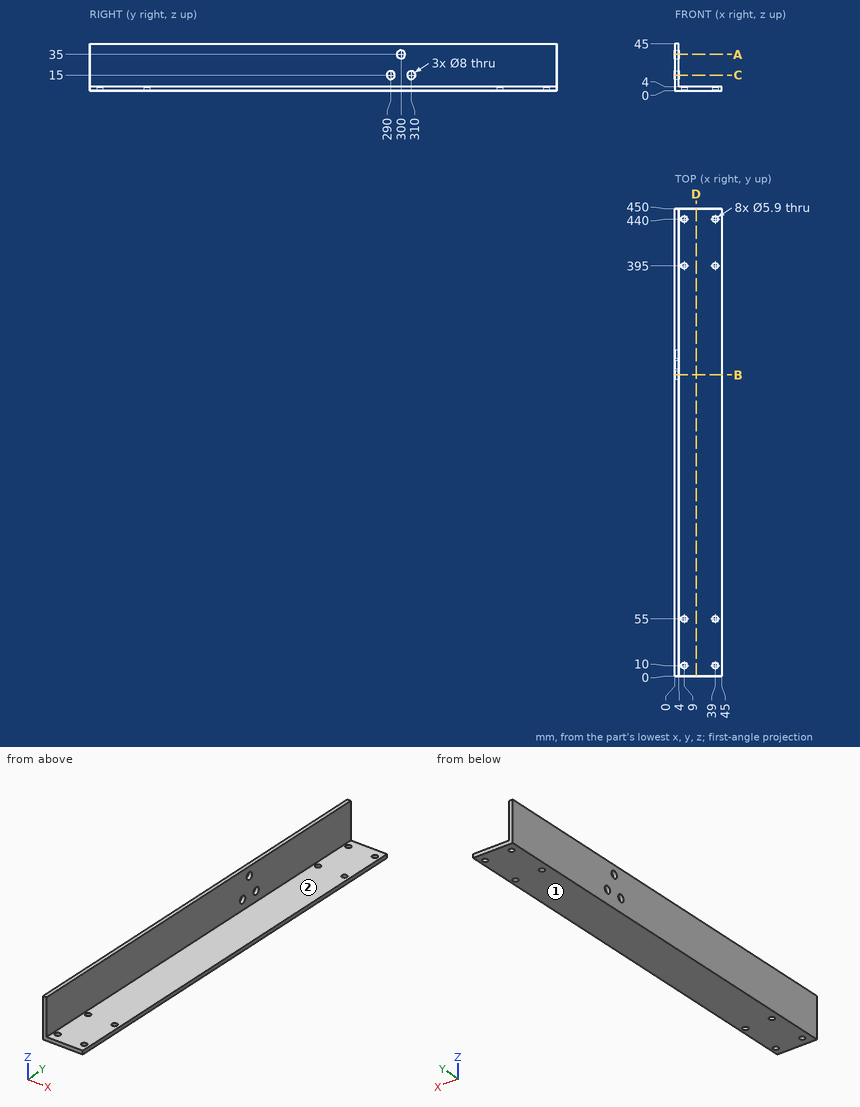
Part print with two shaded views. Sizes in mm from the minimum x, y, z corner. A direction names the side the tool comes from. Coordinates: 2 decimals unless noted, no trailing zeros. Order: outer loops, then holes, each group sorted by start corner. A loop starts at its lowest first (then second) coordinate and runs counter-clockwise, first axis right, second up.
(1) Drill centre lines: L1, parallel to Y at x = 9, z = 3; L2, parallel to Y at x = 38, z = 2; L3, parallel to X at y = 79, z = 21. Where is each one in solid material? Low to high.
Solution:
L1: y = 0 to 7.05, 12.95 to 52.05, 57.95 to 392.05, 397.95 to 437.05, 442.95 to 450
L2: y = 0 to 7.22, 12.78 to 52.22, 57.78 to 392.22, 397.78 to 437.22, 442.78 to 450
L3: x = 0 to 4
(2) Saw through at B-B, the plane y = 290. Write the cut outline in (x, z), and give its area (3 significant figures).
Solution:
outline: (0, 0) - (45, 0) - (45, 4) - (4, 4) - (4, 11) - (0, 11) - close; (0, 19) - (4, 19) - (4, 45) - (0, 45) - close
area: 312 mm2
(3) Pin check, flat tips, straight feed: pin 1 Ø8 at (y, z) = (400.5, 20.5) entering from +X; pin 2 Ø12.5 at (x, y) = (18.5, 241.5) entering from +Z; pin 3 Ø6 at (x, y) = (11.5, 82) entering from -Z. Stop position of each tip, or through.
Solution:
pin 1: stops at x = 4
pin 2: stops at z = 4
pin 3: stops at z = 0
(4) Saw through at A-A, the plane z = 35. Write the cut outline in (x, y), and give its area (3 significant figures).
Solution:
outline: (0, 0) - (4, 0) - (4, 296) - (0, 296) - close; (0, 304) - (4, 304) - (4, 450) - (0, 450) - close
area: 1,770 mm2
(5) Saw through at C-C, the plane z = 15. Write the cut outline in (x, y), and give its area (3 significant figures).
Solution:
outline: (0, 0) - (4, 0) - (4, 286) - (0, 286) - close; (0, 294) - (4, 294) - (4, 306) - (0, 306) - close; (0, 314) - (4, 314) - (4, 450) - (0, 450) - close
area: 1,740 mm2
(6) Which spindle directions (+Z, -Z, +X, -X, +Y, -Y) get a long thin tool onto all of the face, cutting with end or side? Do the marked faces 1 and 2. Say none if no direction does.
Solution:
face 1: -Z, +X, -X, +Y, -Y
face 2: +Z, +X, +Y, -Y
(7) Saw through at D-D, the plane x = 20.5. Write the cut outline in (y, z).
Solution:
outline: (0, 0) - (450, 0) - (450, 4) - (0, 4) - close
